Input: part model. Units: mm. Frame: model coordinates. A direction names the side the tool comes from. Coordinates: 2 decimals unless noted, no trailing zeros. Order: outer loops, then holes, each group sorted by start corner. A loop starts at its lowest first (then second) coordinate and runs counter-clockwise, first axis right, second up. Notation, with made-up numbers: (-21.75, 75) - (35.25, 75) arc R28 cw to (35.25, 112) - close; hole circle Ø3 at (-1, 44). An arc over 180 degrees is marked (long way). One line per question, with ' | ' between items. Start each with the question number.
```python
from build123d import *

# Parameters (mm, degrees)
SKETCH1_R           = 3.9
BOSS_EXTRUDE1_DEPTH = 4.7
CUT_EXTRUDE1_DEPTH  = 3.2


# Read off the part's stored shape, not the designer's step: M5x0.8 Machine Threads Stud1
with BuildPart() as part:
    # Sketch1 → Boss-Extrude1 (new body)
    with BuildSketch(Plane.XY):
        Circle(SKETCH1_R)
    extrude(amount=BOSS_EXTRUDE1_DEPTH)

    # M5x0.8 Machine Threads Stud1 outline → M5x0.8 Machine Threads Stud1 (revolve)
    with BuildSketch(Plane.XZ):
        Polygon((0, 0), (0, -20), (2.055, -20), (2.5, -19.555), (2.5, 0), align=None)
    revolve(axis=Axis((0, 0, 0), (0, 0, 1)))

    # Sketch5 → Cut-Extrude1 (cut)
    with BuildSketch(Plane.XY.offset(4.7)):
        Polygon((1.368919171, -1.859944525), (2.295218794, 0.255546515), (0.926299623, 2.11549104), (-1.368919171, 1.859944525), (-2.295218794, -0.255546515), (-0.926299623, -2.11549104), align=None)
    extrude(amount=-CUT_EXTRUDE1_DEPTH, mode=Mode.SUBTRACT)


solid = part.part
```
(1) Pin query (flat end, axial travel): pin 1 (3 mm diameter, centred on x = -2, z = -6, fed in from +Y); pin 2 (2 mm diameter, centred on x = -0.5, y = -0.5, fed in from +Z); pin 3 (1 mm diameter, centred on y = 0.5, z = -12, fed in from +X). Return the tip coordinate at first contact, or that it passes through.
(2) Section B-B (x = 0). Output: boundary loops of the cut face in (y, z) (3 decimals), then the cut area to 3 significant figures.
(3) Material intervals for line 1 along Y through (x, z) = (-1, -16.5); line 2 along Z through (x, y) = (0.75, -1.25); line 3 along Y through (x, z) = (0, -3.25), sorted ascending. Write a range as from..to.
(4) Reachability of faces 1 (the face through (0, 0, -20)), 2 (the face through (-0.54, -2.44, -9.64)), 3 (the face through (-0.21, 1.99, 3.12)) from +Z, -Z, +X, -X, +Y, -Y: full face, straight path, thin tool, end or side. Return the list, or none.
(5) Section A-A (y = 0). Output: boundary loops of the cut face in (x, z) (3 decimals).
(6) Section C-C (z = -4.75). Output: boundary loops of the cut face in (x, y).
(7) Draft query along Y for faces 4 (the face through (-2.87, 2.64, 2.32)), 5 (the face through (0, 0, 1.5)), 6 (the face through (-2, 1, 4.7)). Return one class per face: +Y half, -Y half, draft (parallel to the pull), parting line (faces both ways), or undercut.
(8) Section D-D (y = -3.25). Output: boundary loops of the cut face in (x, z), then the cut area to 3 significant figures.
Worked answers:
1) pin 1: stops at y = 2.45 | pin 2: stops at z = 1.5 | pin 3: stops at x = 2.5
2) outline: (-3.9, 0) - (-2.5, 0) - (-2.5, -19.555) - (-2.055, -20) - (2.055, -20) - (2.5, -19.555) - (2.5, 0) - (3.9, 0) - (3.9, 4.7) - (2.012, 4.7) - (2.012, 1.5) - (-2.012, 1.5) - (-2.012, 4.7) - (-3.9, 4.7) - close | area: 124 mm²
3) line 1: y = -2.29..2.29 | line 2: z = -20..1.5 | line 3: y = -2.5..2.5
4) face 1: -Z, +X, -X, +Y, -Y | face 2: -Z | face 3: +Z
5) outline: (-3.9, 0) - (-2.5, 0) - (-2.5, -19.555) - (-2.055, -20) - (2.055, -20) - (2.5, -19.555) - (2.5, 0) - (3.9, 0) - (3.9, 4.7) - (2.183, 4.7) - (2.183, 1.5) - (-2.183, 1.5) - (-2.183, 4.7) - (-3.9, 4.7) - close
6) outline: circle Ø5 at (0, 0)
7) face 4: parting line | face 5: undercut | face 6: draft
8) outline: (-2.16, 0) - (2.16, 0) - (2.16, 4.7) - (-2.16, 4.7) - close | area: 20.3 mm²
